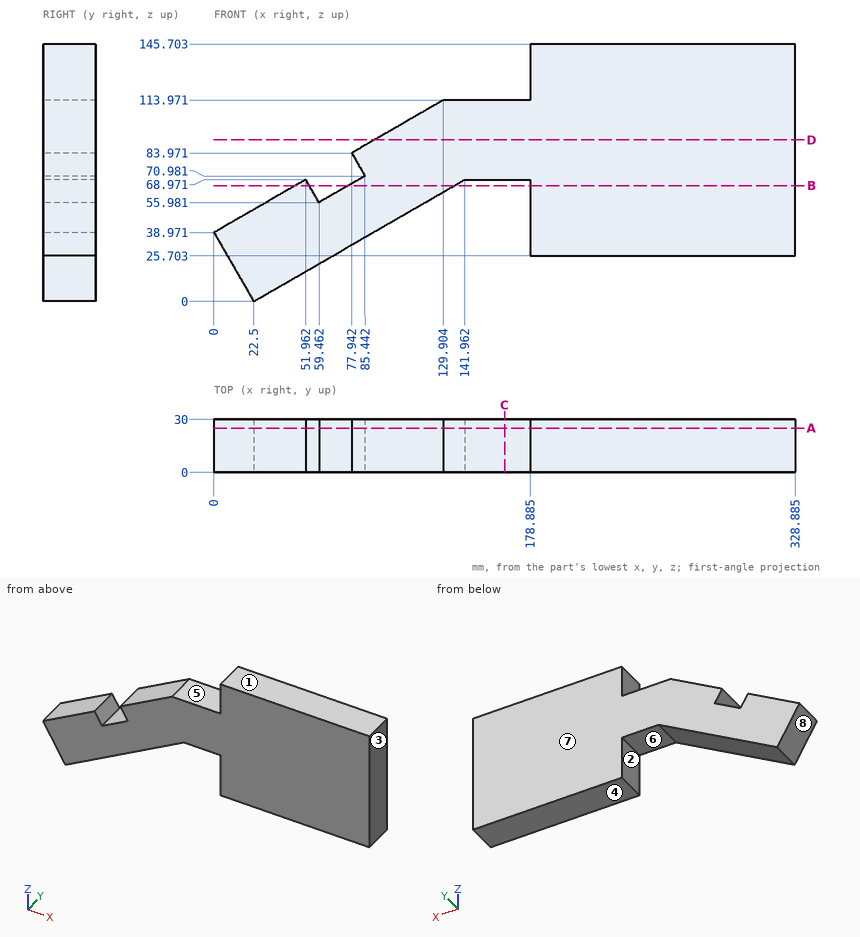
Geometry check sheet. Reference: drawing and pictorial views, mm from the part's lowest x, y, z. A direction names the side the tool comes from. Give positions to 0.01 mm unless a question says otherwise; leave off trailing zeros. Order: outer loops, then holes, each group sorted by start corner. A loop starts at its lowest first (then second) coordinate and runs counter-clockwise, first axis right, second up.
1. Gauge pin test, flat ends, axial feed: pin 1 Ø4 at (x, y) = (125.5, 9) entering from +Z; pin 2 Ø9 at (y, z) = (8, 39) entering from -X; pin 3 Ø2 at (x, y) = (171, 24) entering from -Z. Record the tip position at first contact, or that the pin passes through.
2. Section check B-B, the plane z = 65.5. Give the number of separate pieces and of enclosed holes in the cut face, and give its area (3 significant figures).
3. Thickness scan on L1, parallel to Z at x = 186.5, y = 28.5; L2, parallel to X at y = 10.5, z = 119.5 (1 decimal); L3, parallel to Z at x = 161, y = 12.75. Record the ranges inside material, lowest first.
4. Section check A-A, the plane y = 25. Enter the section's corners in (x, z) (1 decimal).
5. Section check C-C, the plane x = 164.5. Enter the section's corners in (y, z), and give its area (3 significant figures).
6. Release check for a two-part mould opening along X. For the marked faces 1, 2 and 3 record: pulls with the +X half, pulls with the -X half, needs draft (parallel to the pull), parting line crosses it, or undercut.
7. Section check D-D, the plane z = 91.5. Enter the section's corners in (x, y) (1 decimal).
8. Access from +Z, -Z, +X, -X, +Y, -Y to the whole of each face (thin tool, end or side, straight path). Record for the marked faces 4, 5, 6, 7 and 8.
Values follow:
1. pin 1: stops at z = 112.58
1. pin 2: stops at x = 0
1. pin 3: stops at z = 68.97
2. separate pieces: 3
2. enclosed holes: 0
2. area: 6,540 mm2
3. L1: z = 25.7 to 145.7
3. L2: x = 178.9 to 328.9
3. L3: z = 68.97 to 113.97
4. outline: (0, 39) - (22.5, 0) - (142, 69) - (178.9, 69) - (178.9, 25.7) - (328.9, 25.7) - (328.9, 145.7) - (178.9, 145.7) - (178.9, 114) - (129.9, 114) - (77.9, 84) - (85.4, 71) - (59.5, 56) - (52, 69) - close
5. outline: (0, 68.97) - (30, 68.97) - (30, 113.97) - (0, 113.97) - close
5. area: 1,350 mm2
6. face 1: needs draft
6. face 2: undercut
6. face 3: pulls with the +X half
7. outline: (91, 0) - (328.9, 0) - (328.9, 30) - (91, 30) - close
8. face 4: -Z, +X, +Y, -Y
8. face 5: +Z, -X, +Y, -Y
8. face 6: -Z, +Y, -Y
8. face 7: +Z, -Z, +X, -X, +Y
8. face 8: -Z, -X, +Y, -Y
